Here's how the part is built. I have some questions about the finished solid (model axes, mm). A direction names the side the tool comes from. Give positions to 0.01 mm unless a question says otherwise; leave off trailing zeros. Loops run counter-clockwise (first coordinate to the right, second up) from the corner with the lowest first, then second, coordinate; pieces in that order, holes last. Notation, with made-up numbers: (27, 84.5) - (32, 84.5) arc R20 ccw to (32, 100.5) - close; hole circle Ø6 at (-10.5, 3.25). An arc over 180 degrees is marked (long way). Return JSON: item names as keys, results as strings. Group by question number.
(1) I need wall thicknesses on probe 1 along X at (y, z) = (-0.75, 7.5); probe 2 along Z at (x, y) = (-3.75, 2.75); probe 3 along Y at (x, z) = (0, 13). Which ranges of each line are inside material? Lowest first, please. Write a range as [from, to].
(2) If we section it at A-A (z = 13): Please give me the cut outline in (x, y), then the cut area to 3 significant figures.
(3) If we section it at C-C (z = 4.75): Please give me the cut outline in (x, y).
(4) If we section it at B-B (y = 4): Please give me the cut outline in (x, z), then the cut area to 3 significant figures.
(5) On a 3-axis mill with a long thin cutter (end or side, diameter ignored), from which of +Z, -Z, +X, -X, +Y, -Y can I reach the whole of each face in a straight line? I mean faces 1 (the flat face through (-1.2, 1.2, 16)), 2 (the flat face through (-0.1, -3.3, 6)), 3 (the flat face through (0, 0, 6)). Say none if no direction works.
(6) If we section it at D-D (x = 3.5): Please give me the cut outline in (y, z), then the cut area to 3 significant figures.
(7) For P1, Ø4, axis at x = 1, z = 2.5, coming from the +Y side; P2, Ø3, axis at y = 3, z = 10.5, coming from the +X side; P3, Ø1.5, axis at x = -2, z = 13.5, coming from the +Y side, each with a flat end and sliding along its axis, tell me the tip position at first contact or that it passes through.
```python
from build123d import *

# Parameters (mm, degrees)
ESQUISSE1_R             = 3.15
BOSS_EXTRU_1_DEPTH      = 6
ESQUISSE3_R             = 5
BOSS_EXTRU_2_DEPTH      = 10
ESQUISSE4_R             = 1.5
ENL_V_MAT_EXTRU_1_DEPTH = 10
CONG_1_R                = 2


with BuildPart() as part:
    # Esquisse1 → Boss.-Extru.1 (new body)
    with BuildSketch(Plane.XY):
        Circle(ESQUISSE1_R)
    extrude(amount=BOSS_EXTRU_1_DEPTH)

    # Esquisse3 → Boss.-Extru.2 (add)
    with BuildSketch(Plane.XY.offset(6)):
        Circle(ESQUISSE3_R)
    extrude(amount=BOSS_EXTRU_2_DEPTH)

    # Esquisse4 → Enlèv. mat.-Extru.1 (cut)
    with BuildSketch(Plane.XY.offset(16)):
        Circle(ESQUISSE4_R)
    extrude(amount=-ENL_V_MAT_EXTRU_1_DEPTH, mode=Mode.SUBTRACT)

    # Congé1
    cong_1_edges = [part.edges().sort_by_distance(p)[0] for p in [
        (-3.15, 0, 0),
    ]]
    fillet(cong_1_edges, radius=CONG_1_R)


solid = part.part
```
Values:
{
 "1": {"probe 1": "[-4.94, -1.3], [1.3, 4.94]", "probe 2": "[6, 16]", "probe 3": "[-5, -1.5], [1.5, 5]"},
 "2": {"outline": "circle Ø10 at (0, 0); hole circle Ø3 at (0, 0)", "area": "71.5 mm2"},
 "3": {"outline": "circle Ø6.3 at (0, 0)"},
 "4": {"outline": "(-3, 6) - (3, 6) - (3, 16) - (-3, 16) - close", "area": "60.0 mm2"},
 "5": {"face 1": "+Z, +X, -X, +Y, -Y", "face 2": "-Z", "face 3": "+Z"},
 "6": {"outline": "(-3.57, 6) - (3.57, 6) - (3.57, 16) - (-3.57, 16) - close", "area": "71.4 mm2"},
 "7": {"P1": "y = 3.15", "P2": "x = 4.77", "P3": "y = 4.84"}
}
